Part model, mm, in its own coordinate system. Face numbers are marked on the shaded views. A direction names the side the tool comes from. Coordinates: 2 decimals unless noted, no trailing zeros. Loops run counter-clockwise (first coordinate to the right, second up) from the corner with the lowest first, then second, coordinate; pieces in that order, holes last. Notation, with made-up numbers: (43.25, 56) -> (54.25, 56) arc R21 cw to (54.25, 92) -> close; hole circle Ø11 at (18.5, 25.25). An arc over 180 degrees is marked (long way). One line per item, written item: value. Start each with the question number.
from build123d import *

# Parameters (mm, degrees)
F1_DEPTH      = 5
F1_TAPER      = 1
F1_DEPTH_BACK = 5
F1_TAPER_BACK = -1
F3_DEPTH      = 4
F3_DEPTH_BACK = 4


with BuildPart() as f1:
    # F0 (on Front) → F1 (new body, two sides)
    with BuildSketch(Plane.XZ) as f1_sk:
        with BuildLine():
            Line((-4.25, 0), (-2.5, 0))
            ThreePointArc((-2.5, 0), (0, 2.5), (2.5, 0))
            Line((2.5, 0), (4.25, 0))
            Line((4.25, 0), (4.25, 6.75))
            ThreePointArc((4.25, 6.75), (3.8838834765, 7.6338834765), (3, 8))
            Line((3, 8), (-3, 8))
            ThreePointArc((-3, 8), (-3.8838834765, 7.6338834765), (-4.25, 6.75))
            Line((-4.25, 6.75), (-4.25, 0))
        make_face()
    extrude(amount=F1_DEPTH, taper=F1_TAPER)
    extrude(f1_sk.sketch, amount=-F1_DEPTH_BACK, taper=F1_TAPER_BACK)

    # F2 (on Front) → F3 (cut, two sides)
    with BuildSketch(Plane.XZ) as f3_sk:
        with BuildLine():
            Line((6.4694641293, 1.040801663), (7.544499329, 1.8698255615))
            ThreePointArc((7.544499329, 1.8698255615), (0.598902995, 4.9474672346), (-6.4549577741, 2.1267873604))
            Line((-6.4549577741, 2.1267873604), (-5.4162036647, 1.2539537409))
            ThreePointArc((-5.4162036647, 1.2539537409), (0.5705742402, 3.5977590678), (6.4694641293, 1.040801663))
        make_face()
    extrude(amount=-F3_DEPTH, mode=Mode.SUBTRACT)
    extrude(f3_sk.sketch, amount=F3_DEPTH_BACK, mode=Mode.SUBTRACT)


solid = f1.part
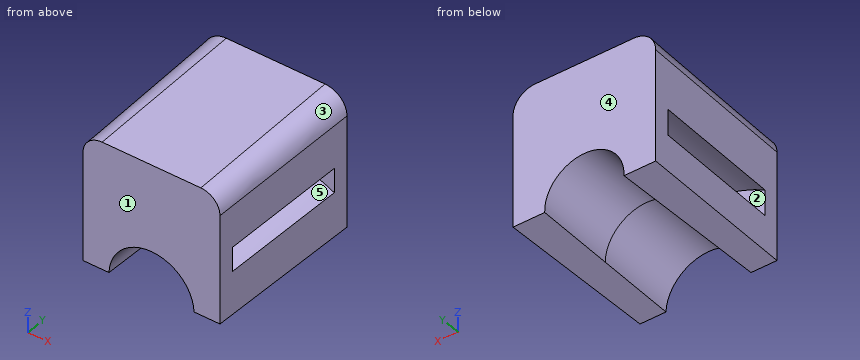
1) Probe line 1 (Y direction, x = -1.5, z = 3.75); line 2 (Z direction, x = -1.25, y = 1.25); line 3 (Z direction, x = 0, y = 2.5). List the from-to ranges inside material, lowest first. Write a range as from..to.
2) Tool access for the marked faces 1 and 2: list every direction of +Z, -Z, +X, -X, +Y, -Y with a clear straight run to the whole face (end or side of a thin tool).
3) Slice it at A-A (z = 5.75). Give the cut face in (x, y), then the cut area to 3 significant figures.
4) Pull direction Z, two halves, no side cores. Call the marked faces 3, 4 and 5: +Z half, -Z half, draft (parallel to the pull), parting line (faces both ways), or undercut.
5) Pin check, flat tips, straight feed: pin 1 Ø3 at (y, z) = (2.5, 6.5) entering from -X; pin 2 Ø3 at (x, y) = (-0.5, -4) entering from -Z; pin 3 Ø5 at (x, y) = (-1.5, 0.5) entering from +Z. Stop position of each tip, or through.
Check sheet entries:
1. line 1: y = -5..-4, 4..5
1. line 2: z = 2.14..3.43, 4.81..8.02
1. line 3: z = 2.46..3.59, 4.94..8.04
2. face 1: +Z, -Z, +X, -X, -Y
2. face 2: none
3. outline: (-4.34, 5) -> (-4.16, -5) -> (4.16, -5) -> (4.34, 5) -> close
3. area: 85.0 mm^2
4. face 3: +Z half
4. face 4: draft
4. face 5: undercut
5. pin 1: stops at x = -4.32
5. pin 2: stops at z = 1.61
5. pin 3: stops at z = 8.05
